from build123d import *

# Parameters (mm, degrees)
ESQUISSE2_R             = 3
ESQUISSE2_W             = 60
ESQUISSE2_H             = 25
BOSS_EXTRU_2_DEPTH      = 5
ESQUISSE3_W             = 50
ESQUISSE3_H             = 10
ENL_V_MAT_EXTRU_1_DEPTH = 2.5
ESQUISSE4_W             = 50
ESQUISSE4_H             = 6
ENL_V_MAT_EXTRU_2_DEPTH = 159.049070395
ESQUISSE5_W             = 30
ESQUISSE5_H             = 20
ENL_V_MAT_EXTRU_3_DEPTH = 4
CHANFREIN1_SIZE         = 2
ESQUISSE6_R             = 4
ENL_V_MAT_EXTRU_4_DEPTH = 4
ESQUISSE7_R             = 3
ENL_V_MAT_EXTRU_5_DEPTH = 159.049070395
ESQUISSE8_R             = 2
ENL_V_MAT_EXTRU_6_DEPTH = 158.989742239
CONG_2_R                = 3
ESQUISSE9_R             = 10.1
ESQUISSE9_R_2           = 1.5
ENL_V_MAT_EXTRU_7_DEPTH = 159.049070395


with BuildPart() as part:
    # Esquisse2 → Boss.-Extru.2 (new body)
    with BuildSketch(Plane.XY):
        Polygon((-40, 10), (-25, 10), (-25, 0), (25, 0), (25, 10), (40, 10), (40, 52), (116.213203436, 52), (116.213203436, 85.786796564), (95, 107), (-95, 107), (-116.213203436, 85.786796564), (-116.213203436, 52), (-40, 52), align=None)
        with Locations((-30, 63)):
            Circle(ESQUISSE2_R, mode=Mode.SUBTRACT)
        with Locations((-30, 22)):
            Circle(ESQUISSE2_R, mode=Mode.SUBTRACT)
        with Locations((30, 22)):
            Circle(ESQUISSE2_R, mode=Mode.SUBTRACT)
        with Locations((30, 63)):
            Circle(ESQUISSE2_R, mode=Mode.SUBTRACT)
        with Locations((0, 39.5)):
            Rectangle(ESQUISSE2_W, ESQUISSE2_H, mode=Mode.SUBTRACT)
    extrude(amount=BOSS_EXTRU_2_DEPTH)

    # Esquisse3 → Enlèv. mat.-Extru.1 (cut)
    with BuildSketch(Plane.XY.offset(5)):
        with Locations((0, 5)):
            Rectangle(ESQUISSE3_W, ESQUISSE3_H)
    extrude(amount=-ENL_V_MAT_EXTRU_1_DEPTH, mode=Mode.SUBTRACT)

    # Esquisse4 → Enlèv. mat.-Extru.2 (cut, through all)
    with BuildSketch(Plane.XY.offset(5)):
        with Locations((0, 98)):
            Rectangle(ESQUISSE4_W, ESQUISSE4_H)
    extrude(amount=-ENL_V_MAT_EXTRU_2_DEPTH, mode=Mode.SUBTRACT)

    # Esquisse5 → Enlèv. mat.-Extru.3 (cut)
    with BuildSketch(Plane.XY.offset(5)):
        with Locations((0, 80)):
            Rectangle(ESQUISSE5_W, ESQUISSE5_H)
    extrude(amount=-ENL_V_MAT_EXTRU_3_DEPTH, mode=Mode.SUBTRACT)

    # Chanfrein1
    chanfrein1_edges = [part.edges().sort_by_distance(p)[0] for p in [
        (-33, 63, 0),
        (-33, 22, 0),
        (27, 22, 0),
        (27, 63, 0),
    ]]
    chamfer(chanfrein1_edges, length=CHANFREIN1_SIZE - 0.0001)  # a hair under: the kernel refuses the full size

    # Esquisse6 → Enlèv. mat.-Extru.4 (cut)
    with BuildSketch(Plane.XY.offset(5)):
        with Locations((-40.5, 96)):
            Circle(ESQUISSE6_R)
        with Locations((40.5, 96)):
            Circle(ESQUISSE6_R)
    extrude(amount=-ENL_V_MAT_EXTRU_4_DEPTH, mode=Mode.SUBTRACT)

    # Esquisse7 → Enlèv. mat.-Extru.5 (cut, through all)
    with BuildSketch(Plane.XY.offset(5)):
        with Locations((-85, 97)):
            Circle(ESQUISSE7_R)
        with Locations((85, 97)):
            Circle(ESQUISSE7_R)
    extrude(amount=-ENL_V_MAT_EXTRU_5_DEPTH, mode=Mode.SUBTRACT)

    # Esquisse8 → Enlèv. mat.-Extru.6 (cut, through all)
    with BuildSketch(Plane.XY.offset(2.5)):
        with Locations((-15, 4)):
            Circle(ESQUISSE8_R)
        with Locations((15, 4)):
            Circle(ESQUISSE8_R)
    extrude(amount=-ENL_V_MAT_EXTRU_6_DEPTH, mode=Mode.SUBTRACT)

    # Congé2
    cong_2_edges = [part.edges().sort_by_distance(p)[0] for p in [
        (30, 52, 2.5),
        (-30, 27, 2.5),
        (30, 27, 2.5),
        (-25, 95, 2.5),
        (25, 95, 2.5),
        (25, 101, 2.5),
        (-25, 101, 2.5),
        (-30, 52, 2.5),
        (116.213203436, 52, 2.5),
        (-40, 10, 2.5),
        (40, 10, 2.5),
        (-116.213203436, 52, 2.5),
        (-15, 90, 3),
        (-15, 70, 3),
        (15, 70, 3),
        (15, 90, 3),
        (40, 52, 2.5),
        (-40, 52, 2.5),
        (-25, 10, 1.25),
        (25, 10, 1.25),
        (25, 0, 1.25),
        (-25, 0, 1.25),
    ]]
    fillet(cong_2_edges, radius=CONG_2_R - 0.0001)  # a hair under: the kernel refuses the full size

    # Esquisse9 → Enlèv. mat.-Extru.7 (cut, through all)
    with BuildSketch(Plane.XY.offset(5)):
        with Locations((100.513203436, 67.7)):
            Circle(ESQUISSE9_R)
        with Locations((113.213203436, 67.7)):
            Circle(ESQUISSE9_R_2)
        with Locations((100.513203436, 80.4)):
            Circle(ESQUISSE9_R_2)
        with Locations((87.813203436, 67.7)):
            Circle(ESQUISSE9_R_2)
        with Locations((100.513203436, 55)):
            Circle(ESQUISSE9_R_2)
        with Locations((-100.513203436, 67.7)):
            Circle(ESQUISSE9_R)
        with Locations((-87.813203436, 67.7)):
            Circle(ESQUISSE9_R_2)
        with Locations((-100.513203436, 80.4)):
            Circle(ESQUISSE9_R_2)
        with Locations((-113.213203436, 67.7)):
            Circle(ESQUISSE9_R_2)
        with Locations((-100.513203436, 55)):
            Circle(ESQUISSE9_R_2)
    extrude(amount=-ENL_V_MAT_EXTRU_7_DEPTH, mode=Mode.SUBTRACT)


solid = part.part
Check sheet for the modelled part. Datum: model origin and axes. Units: mm. A direction names the side the tool comes from. Round coordinates to 2 decimals unless told otherwise and drop trailing zeros. Loops run counter-clockwise (first coordinate to the right, second up) from the corner with the lowest first, then second, coordinate; pieces in that order, holes last. Notation, with made-up numbers: (47.25, 34.25) - (92.25, 34.25) arc R29 cw to (92.25, 65.25) - close; hole circle Ø10 at (54.5, 25). An arc over 180 degrees is marked (long way). Answer as CSV lines item,"result". Start each with the question number.
Item 1: Section check C-C (y = 33). Record the boundary of the cut face in (x, z), and give its area (3 significant figures).
Item 2: Scan lines: line 1 (Y direction, x = 17.5, z = 1.5); line 2 (Y direction, x = 7, z = 1.8); line 3 (X direction, y = 30, z = 1). Record each from-to range of solid material in increasing order. Write a range as [from, to].
Item 3: Release check for a two-part mould opening along Y. For faces 4 (the cylindrical face through (27, 22, 3)), 5 (the flat face through (0, 5, 2.5)), 6 (the flat face through (78, 52, 2)) record: +Y half, -Y half, draft (parallel to the pull), parting line (faces both ways), or undercut.
Item 4: Section check D-D (z = 3.6). Count the separate pieces of the cut face and the enclosed holes in it, and give its area (3 significant figures).
Item 5: Section check B-B (y = 63). Record the boundary of the cut face in (x, z).
Item 6: Section check A-A (x = 1.5). Record the boundary of the cut face in (y, z), and give its area (3 significant figures).
Item 7: Depth check by flat-ended pin: P1, Ø1, axis at x = -81.5, z = 2.5, coming from the -Y side; P2, Ø1.5, axis at y = 41, z = 1.5, coming from the -X side; P3, Ø3, axis at y = 34.5, z = 2.5, coming from the +X side. Enter the tip coordinate at first touch or a pass-through.
Item 8: Set-up check for faces 1 (the flat face through (106, 96, 2)), 2 (the flat face through (30, 39, 2)), 3 (the flat face through (-15, 80, 3)): record each of +Z, -Z, +X, -X, +Y, -Y from which the full face is reachable in a straight line by a thin tool's end or side.
Report:
1,outline,"(-40, 0) - (-30, 0) - (-30, 5) - (-40, 5) - close; (30, 0) - (40, 0) - (40, 5) - (30, 5) - close"
1,area,"100 mm2"
2,line 1,"y = [0, 27], [52, 95], [101, 107]"
2,line 2,"y = [0, 27], [52, 70], [90, 95], [101, 107]"
2,line 3,"x = [-40, -30], [30, 40]"
3,face 4,"undercut"
3,face 5,"draft"
3,face 6,"-Y half"
4,separate pieces,"1"
4,enclosed holes,"21"
4,area,"12,300 mm2"
5,outline,"(-116.21, 0) - (-109.45, 0) - (-109.45, 5) - (-116.21, 5) - close; (-91.57, 0) - (-35, 0) - (-33, 2) - (-33, 5) - (-91.57, 5) - close; (-27, 2) - (-25, 0) - (25, 0) - (27, 2) - (27, 5) - (-27, 5) - close; (33, 2) - (35, 0) - (91.57, 0) - (91.57, 5) - (33, 5) - close; (109.45, 0) - (116.21, 0) - (116.21, 5) - (109.45, 5) - close"
6,outline,"(0, 0) - (27, 0) - (27, 5) - (10, 5) - (10, 2.5) - (0, 2.5) - close; (52, 0) - (95, 0) - (95, 5) - (90, 5) - (90, 1) - (70, 1) - (70, 5) - (52, 5) - close; (101, 0) - (107, 0) - (107, 5) - (101, 5) - close"
6,area,"275 mm2"
7,P1,"stops at y = 52"
7,P2,"stops at x = -40"
7,P3,"stops at x = 40"
8,face 1,"+Z, -Z, +X, +Y"
8,face 2,"+Z, -Z"
8,face 3,"+Z"
